Source: CAD feature listing. Evaluate the final solid. Frame: model axes, mm. Give positions to 0.01 mm unless a question says otherwise; leave off trailing zeros. Order: outer loops, then holes, each group sorted by start corner. A loop starts at its lowest first (then second) coordinate and runs counter-clockwise, first axis right, second up.
1) Section B-B, the plane x = 0. Return loops of the section in (y, z), plus the area to 3 significant figures.
2) Material intervals for line 1 (Y direction, x = 0, z = 1.25); line 2 (X direction, y = -37, z = 1.3); line 3 (X direction, y = -33.5, z = 2.3), sorted ascending.
3) First-contact query: P1, Ø1.5, axis at y = 37, z = 2, coming from the -X side; P2, Ø9, axis at x = 0, y = 69.85, coming from the +Z side (3 decimals); P3, Ø1, axis at y = 44, z = 1, coming from the +X side. Flat tips, straight axial feed; report the tip coordinate or a pass-through.
4) Section C-C, the plane z = 1.9. Give the number of separate pieces and of enclosed holes in the cut face, plus the area to 3 significant figures.
```python
from build123d import *

# Parameters (mm, degrees)
F0_W     = 96.52
F0_H     = 165.1
F0_R     = 4.1275
F0_R_2   = 7.3025
F1_DEPTH = 2.54
F2_SIZE  = 2.53999


# Not quite as in the source:
# - a fillet or chamfer is up to 0.001 mm smaller than in the source, because OpenCascade refuses the exact size


with BuildPart() as f1:
    # F0 (on Top) → F1 (new body)
    with BuildSketch(Plane.XY):
        Rectangle(F0_W, F0_H)
        with Locations((0, 55.245)):
            Circle(F0_R, mode=Mode.SUBTRACT)
        with Locations((0, 69.85)):
            Circle(F0_R_2, mode=Mode.SUBTRACT)
    extrude(amount=F1_DEPTH)

    # F2 (size 2.54 in the source; OpenCascade refuses exactly that, so slightly less here)
    f2_edges = [f1.edges().sort_by_distance(p)[0] for p in [
        (-48.26, 0, 0),
        (48.26, 0, 0),
    ]]
    chamfer(f2_edges, length=F2_SIZE)


solid = f1.part
```
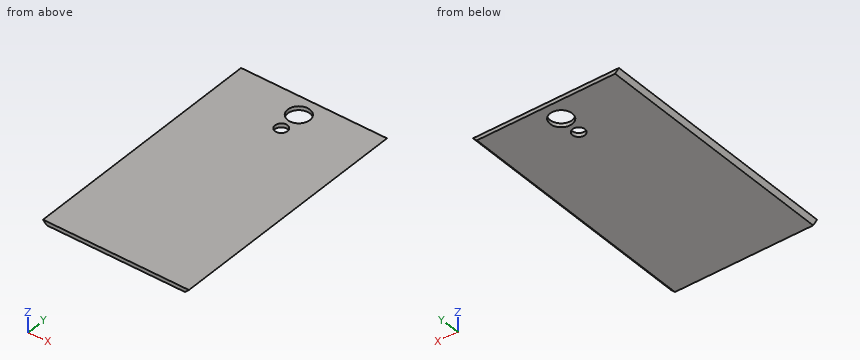
From the geometry:
1. outline: (-82.55, 0) - (51.12, 0) - (51.12, 2.54) - (-82.55, 2.54) - close; (59.37, 0) - (62.55, 0) - (62.55, 2.54) - (59.37, 2.54) - close; (77.15, 0) - (82.55, 0) - (82.55, 2.54) - (77.15, 2.54) - close
1. area: 361 mm2
2. line 1: y = -82.55 to 51.12, 59.37 to 62.55, 77.15 to 82.55
2. line 2: x = -47.02 to 47.02
2. line 3: x = -48.02 to 48.02
3. P1: stops at x = -48.26
3. P2: passes through
3. P3: stops at x = 47.22
4. separate pieces: 1
4. enclosed holes: 2
4. area: 15,500 mm2
